from build123d import *

# Parameters (mm, degrees)
RADDURCHMESSER_R                = 350
AUFSATZ_LINEAR_AUSTRAGEN1_DEPTH = 117.5
AUFSATZ_LINEAR_AUSTRAGEN2_DEPTH = 117.5
KREISMUSTER1_COUNT              = 20


with BuildPart() as part:
    # Raddurchmesser → Aufsatz-Linear austragen1 (new body, symmetric)
    with BuildSketch(Plane.XY):
        Circle(RADDURCHMESSER_R)
    extrude(amount=AUFSATZ_LINEAR_AUSTRAGEN1_DEPTH, both=True)

    # Schaufelschnitt → Aufsatz-Linear austragen2 (add, symmetric)
    with BuildSketch(Plane.XY):
        Polygon((122.625257529, 327.815567379), (120.693405876, 328.333205469), (137.000570821, 389.192373572), (53.213617667, 472.979326726), (-0.845236523, 498.187384426), (0, 500), (54.378467222, 474.642904296), (139.231280965, 389.790090553), align=None)
    aufsatz_linear_austragen2 = extrude(amount=AUFSATZ_LINEAR_AUSTRAGEN2_DEPTH, both=True)

    # Kreismuster1: Aufsatz-Linear austragen2 ×20 about axis
    kreismuster1_axis = Axis((0, 0, 0), (0, 0, 1))
    for i in range(1, KREISMUSTER1_COUNT):
        add(aufsatz_linear_austragen2.rotate(kreismuster1_axis, i * 360 / KREISMUSTER1_COUNT))


solid = part.part
The model under review builds one solid part; all positions refer to its coordinate system, in mm. A direction names the side the tool comes from. Give positions to 0.01 mm unless a question says otherwise; leave off trailing zeros. Order: outer loops, then holes, each group sorted by start corner. A loop starts at its lowest first (then second) coordinate and runs counter-clockwise, first axis right, second up. Notation, with made-up numbers: M 13,55 L 41,55 A18 ccw 41,66 Z; hole C 30,58 d1. An arc over 180 degrees is marked long. Use one line per item in the form item = value. Start each with the question number.
Item 1: For faces 4 (the flat face through (292.03, -330.46, 1.64)), 5 (the flat face through (-332.236, -293.6, 1.645)), 6 (the flat face through (308.23, 378.64, 1.64)), list the 3-axis set-ups (+Z, -Z, +X, -X, +Y, -Y) from which the entire face can be reached by the end or side of a thin tool; tool diameter is ignored.
Item 2: We need section A-A on y = -168.5. Give the boundary of the cut face in (x, z).
Item 3: To check wall thickness, follow line 1 along X through (y, z) = (-151.5, -78.5); line 2 along X through (y, z) = (34.5, 6.5); line 3 along Y through (x, z) = (-45, 0.5). State the ranges of each line that lie inside material, in increasing order. Write a range as from..to.
Item 4: Insertion check: pin 1 Ø4 at (x, z) = (186, -65.5) entering from +Y; pin 2 Ø1 at (y, z) = (-75, 25.5) entering from -X; pin 3 Ø1.5 at (x, z) = (-220, 0.5) entering from -Y. Each pin has a flat end and moves straight along its axis. Give the tip position at first contact, or say it passes through.
Item 5: The part is to be moulded in two halves that separate along X. For faces 1 (the flat face through (-11.695, -380.674, 1.645)), 2 (the flat face through (487.5, -26.81, 1.64)), 3 (the flat face through (-26.81, -487.5, 1.64)), say which applies: pulls with the +X half, pulls with the -X half, needs draft (parallel to the pull), parting line crosses it, or undercut.
Completed:
q1.face_4 = +Z, -Z
q1.face_5 = +Z, -Z, -Y
q1.face_6 = +Z, -Z, +X, +Y
q2.outline = M -405.43,-117.5 L -403.4,-117.5 L -403.4,117.5 L -405.43,117.5 Z; M -306.77,-117.5 L 306.77,-117.5 L 306.77,117.5 L -306.77,117.5 Z; M 459.75,-117.5 L 462.48,-117.5 L 462.48,117.5 L 459.75,117.5 Z
q3.line_1 = -475.16..-473.14, -402.73..-400.71, -315.51..315.51
q3.line_2 = -483.91..-481.71, -348.3..348.3, 435.17..437.41
q3.line_3 = -479.02..-476.81, -347.1..347.1, 440.52..442.76
q4.pin_1 = 448.03
q4.pin_2 = -458.3
q4.pin_3 = -393.67
q5.face_1 = undercut
q5.face_2 = pulls with the +X half
q5.face_3 = pulls with the -X half
